Design review of the part built by this model. Coordinates are the model's own, in mm. A direction names the side the tool comes from. Coordinates: 2 decimals unless noted, no trailing zeros. Write each loop counter-clockwise with the first axis right and the second up, starting at its lowest first coordinate (ties: lowest second). Pieces come first, ordered by that corner, then holes. Notation, with made-up numbers: M 13,-24.5 L 54,-24.5 A17 cw 54,-9.5 Z; hole C 18.25,-1 d10. An arc over 180 degrees is marked long. Write each question's results on one line, items separated by ' | '. Start each with the question number.
```python
from build123d import *

# Parameters (mm, degrees)
F0_R     = 2.5781
F0_R_2   = 2.57175
F1_DEPTH = 25.4


with BuildPart() as f1:
    # F0 (on Top) → F1 (new body)
    with BuildSketch(Plane.XY):
        with BuildLine():
            ThreePointArc((-31.291722, -68.875), (0, -95.25), (31.291722, -68.875))
            Line((31.291722, -68.875), (41.886557, -7.194882))
            ThreePointArc((41.886557, -7.194882), (0, 42.5), (-41.886557, -7.194882))
            Line((-41.886557, -7.194882), (-31.291722, -68.875))
        make_face()
        with Locations((0, -88.9)):
            Circle(F0_R, mode=Mode.SUBTRACT)
        with Locations((-36.2458, 0)):
            Circle(F0_R, mode=Mode.SUBTRACT)
        with BuildLine():
            ThreePointArc((-29.550596, -5.173228), (0, 30), (29.550596, -5.173228))
            Line((29.550596, -5.173228), (18.764628, -66.785))
            ThreePointArc((18.764628, -66.785), (0, -82.55), (-18.764628, -66.785))
            Line((-18.764628, -66.785), (-29.550596, -5.173228))
        make_face(mode=Mode.SUBTRACT)
        with Locations((36.2458, 0)):
            Circle(F0_R, mode=Mode.SUBTRACT)
        with Locations((0, 36.2458)):
            Circle(F0_R_2, mode=Mode.SUBTRACT)
    extrude(amount=F1_DEPTH)


solid = f1.part
```
Item 1: We need section B-B on x = 0. State the section outline as (y, z) points.
Item 2: For faces 1 (the flat face through (-36.663, -37.603, 12.522)), 2 (the flat face through (-24.082, -36.41, 12.522)), list the 3-axis set-ups (+Z, -Z, +X, -X, +Y, -Y) from which the entire face can be reached by the end or side of a thin tool; tool diameter is ignored.
Item 3: We need section D-D on z = 22.25. Count the separate pieces of the cut face and the enclosed holes in it, then the cut area to 3 significant figures.
Item 4: We need section C-C on y = 0. State the section outline as (x, z) points, then the cut area to 3 significant figures.
Item 5: Draft analysis for pull direction Y (two halves, no side actions). For faces 3 (the flat face through (24.233, -35.548, 12.522)), 4 (the flat face through (-25, -36, 0)), 5 (the flat face through (36.515, -38.467, 12.522)), state which applies: released by +Y, released by -Y, zero draft, split by the parting line, or undercut.
Item 6: Insertion check: pin 1 Ø5 at (y, z) = (-18.5, 21) entering from +X; pin 2 Ø6 at (x, y) = (0, 36.25) entering from +Z; pin 3 Ø1 at (y, z) = (-27.5, 5) entering from +X; pin 4 Ø1.5 at (y, z) = (-66, 4) entering from +X. Each pin has a flat end and moves straight along its axis. Give the tip position at first contact, or say it passes through.
Item 7: Wall thickness on L1, parallel to Y at x = -1, z = 19.75; L2, parallel to Y at x = 2, z = 19.25; L3, parallel to X at y = -75, z = 11.25: over which ranges is each line inside the solid? List them lowest first.
Item 8: We need section A-A on y = -88.9. State the section outline as (x, z) points, then the cut area to 3 significant figures.
Answer:
1) outline: M -95.25,0 L -91.48,0 L -91.48,25.4 L -95.25,25.4 Z; M -86.32,0 L -82.55,0 L -82.55,25.4 L -86.32,25.4 Z; M 30,0 L 33.67,0 L 33.67,25.4 L 30,25.4 Z; M 38.82,0 L 42.5,0 L 42.5,25.4 L 38.82,25.4 Z
2) face 1: +Z, -Z, -X, -Y | face 2: +Z, -Z
3) separate pieces: 1 | enclosed holes: 5 | area: 3,980 mm^2
4) outline: M -42.5,0 L -38.82,0 L -38.82,25.4 L -42.5,25.4 Z; M -33.67,0 L -30,0 L -30,25.4 L -33.67,25.4 Z; M 30,0 L 33.67,0 L 33.67,25.4 L 30,25.4 Z; M 38.82,0 L 42.5,0 L 42.5,25.4 L 38.82,25.4 Z | area: 373 mm^2
5) face 3: undercut | face 4: zero draft | face 5: released by -Y
6) pin 1: stops at x = 40.37 | pin 2: stops at z = 25.4 | pin 3: stops at x = 38.48 | pin 4: stops at x = 31.91
7) L1: y = -95.23 to -91.28, -86.52 to -82.52, 29.98 to 33.88, 38.62 to 42.49 | L2: y = -95.19 to -90.53, -87.27 to -82.44, 29.93 to 34.63, 37.86 to 42.45 | L3: x = -29.59 to -15.19, 15.19 to 29.59
8) outline: M -19.05,0 L -2.58,0 L -2.58,25.4 L -19.05,25.4 Z; M 2.58,0 L 19.05,0 L 19.05,25.4 L 2.58,25.4 Z | area: 837 mm^2
